from build123d import *

# Parameters (mm, degrees)
F0_R     = 12.7
F1_DEPTH = 76.2
F2_R     = 19.05
F3_DEPTH = 5.08
F5_DEPTH = 2.54
F7_DEPTH = 2.54


with BuildPart() as f1:
    # F0 (on Top) → F1 (new body)
    with BuildSketch(Plane.XY):
        Circle(F0_R)
    extrude(amount=-F1_DEPTH)

    # F2 (on Top) → F3 (join)
    with BuildSketch(Plane.XY):
        Circle(F2_R)
    extrude(amount=F3_DEPTH)

    # F4 (on Front) → F5 (join)
    with BuildSketch(Plane.XZ):
        Polygon((-5.08, 0), (0, 0), (0, 114.3), (-5.08, 101.6), align=None)
        Polygon((0, 114.3), (0, 0), (5.08, 0), (5.08, 101.6), align=None)
    extrude(amount=-F5_DEPTH)

    # F6 (on Front) → F7 (join)
    with BuildSketch(Plane.XZ):
        Polygon((-5.08, 0), (0, 0), (0, 114.3), (-5.08, 101.6), align=None)
        Polygon((0, 114.3), (0, 0), (5.08, 0), (5.08, 101.6), align=None)
    extrude(amount=F7_DEPTH)


solid = f1.part
Work out the finished part from the listing and answer in its coordinate system (mm). A direction names the side the tool comes from. Coordinates: 2 decimals unless noted, no trailing zeros. Loops run counter-clockwise (first coordinate to the right, second up) from the corner with the lowest first, then second, coordinate; pieces in that order, holes last. Notation, with made-up numbers: (50, 81.25) -> (105, 81.25) arc R30 cw to (105, 114.25) -> close; hole circle Ø6 at (14, 76). An arc over 180 degrees is marked (long way). Write each question's results on one line, items separated by ' | '. Start each with the question number.
1) Flat-ended cylindrical pins translate along their axes: P1, Ø5, axis at x = 6, y = -13, coming from the -Z side; P2, Ø4, axis at y = 0.5, z = 51.5, coming from the +X side; P3, Ø12, axis at y = -9.5, z = 80.5, coming from the -X side; P4, Ø5, axis at x = -5, y = 9.5, coming from the +Z side. Find the tip coordinate at first contact, or state that the pin passes through.
2) Consider line 1 along Y through (x, z) = (-2.5, 22.5); line 2 along Z through (x, y) = (17.5, 5.5); line 3 along X through (y, z) = (-2, 31.5). Determine where each line is inside the solid, lowest interval first.
3) Find section B-B on x = -11. Determine the outline of the cut face in (y, z).
4) Find section D-D on y = 8. Determine the outline of the cut face in (x, z).
5) Find section C-C on z = 9. Determine the outline of the cut face in (x, y).
6) Find section A-A on y = 0. Determine the outline of the cut face in (x, z), then the cut area to 3 significant figures.
7) For faces 1 (the flat face through (4, -12.4, 0)), 2 (the flat face through (5.08, 0, 53)), 3 (the flat face through (0, -2.54, 60)), 4 (the flat face through (0, 2.54, 60)), determine the directions among +Z, -Z, +X, -X, +Y, -Y from which every point of the face is accessible in a straight line to the end or side of a thin tool.
Response values:
1) P1: stops at z = -76.2 | P2: stops at x = 5.08 | P3: passes through | P4: stops at z = 5.08
2) line 1: y = -2.54 to 2.54 | line 2: z = 0 to 5.08 | line 3: x = -5.08 to 5.08
3) outline: (-15.55, 0) -> (-6.35, 0) -> (-6.35, -76.2) -> (6.35, -76.2) -> (6.35, 0) -> (15.55, 0) -> (15.55, 5.08) -> (-15.55, 5.08) -> close
4) outline: (-17.29, 0) -> (-9.86, 0) -> (-9.86, -76.2) -> (9.86, -76.2) -> (9.86, 0) -> (17.29, 0) -> (17.29, 5.08) -> (-17.29, 5.08) -> close
5) outline: (-5.08, -2.54) -> (5.08, -2.54) -> (5.08, 2.54) -> (-5.08, 2.54) -> close
6) outline: (-19.05, 0) -> (-12.7, 0) -> (-12.7, -76.2) -> (12.7, -76.2) -> (12.7, 0) -> (19.05, 0) -> (19.05, 5.08) -> (5.08, 5.08) -> (5.08, 101.6) -> (0, 114.3) -> (-5.08, 101.6) -> (-5.08, 5.08) -> (-19.05, 5.08) -> close | area: 3,170 mm^2
7) face 1: -Z | face 2: +Z, +X, +Y, -Y | face 3: +Z, +X, -X, -Y | face 4: +Z, +X, -X, +Y
